Source: CAD feature listing. Evaluate the final solid. Frame: model axes, mm. Round coordinates to 2 decimals unless told otherwise and drop trailing zeros. Loops run counter-clockwise (first coordinate to the right, second up) from the corner with the lowest first, then second, coordinate; pieces in that order, holes last. Notation, with made-up numbers: M -28.75,-17 L -1.75,-17 A19 ccw -1.75,-9 Z; hole C 43,52.5 d4. An arc over 180 degrees is marked long. Write each question's results on one line, items separated by ' | '. Start each with the question number.
1. Section C-C on x = 138.5. Output: boundary loops of the cut face in (y, z), and give its area (3 significant figures).
2. Contact query for flat-ended pins moving along their axis: pin 1 Ø0.9 at (y, z) = (160.5, 1) entering from +X; pin 2 Ø10 at (x, y) = (115.5, 150) entering from -Z. Output: stop coordinate, or through.
3. Ray query, line 1 (X direction, y = 117.5, z = 1.8); line 2 (Y direction, x = 141, z = 0.9); line 3 (X direction, y = -16, z = 2.8). Return the intervals inside material, ascending.
4. Section B-B on y = 154.5. Output: boundary loops of the cut face in (x, z).
5. Section A-A on z = 1.85. Output: boundary loops of the cut face in (x, y).
from build123d import *

# Parameters (mm, degrees)
BOSS_EXTRU_1_DEPTH = 3
CHANFREIN1_SIZE    = 40


with BuildPart() as part:
    # Esquisse1 → Boss.-Extru.1 (new body)
    with BuildSketch(Plane.XY):
        Polygon((115.873312648, 190.152785154), (115.873312648, 90.152785154), (160.873312648, 34.730964145), (160.873312648, -41.347214846), (-109.126687352, -41.347214846), (-109.126687352, 34.730964145), (-64.126687352, 90.152785154), (-64.126687352, 190.152785154), align=None)
    extrude(amount=BOSS_EXTRU_1_DEPTH)

    # Chanfrein1
    chanfrein1_edges = [part.edges().sort_by_distance(p)[0] for p in [
        (160.873312648, -41.347214846, 1.5),
        (-109.126687352, -41.347214846, 1.5),
    ]]
    chamfer(chanfrein1_edges, length=CHANFREIN1_SIZE)


solid = part.part
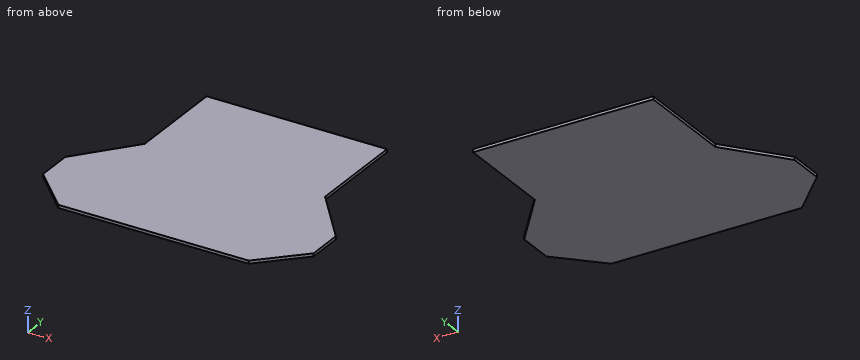
Taken from the geometry:
1) outline: M -23.72,0 L 62.29,0 L 62.29,3 L -23.72,3 Z | area: 258 mm^2
2) pin 1: x = 115.87 | pin 2: z = 0
3) line 1: -64.13 to 115.87 | line 2: -21.22 to 59.21 | line 3: -94.47 to 146.22
4) outline: M -64.13,0 L 115.87,0 L 115.87,3 L -64.13,3 Z
5) outline: M -109.13,-1.35 L -69.13,-41.35 L 120.87,-41.35 L 160.87,-1.35 L 160.87,34.73 L 115.87,90.15 L 115.87,190.15 L -64.13,190.15 L -64.13,90.15 L -109.13,34.73 Z
